from build123d import *

# Parameters (mm, degrees)
ESTRUSIONE_ESTRUSIONE3_DEPTH = 1.5


with BuildPart() as part:
    # Schizzo1 → Estrusione-Estrusione3 (new body, symmetric)
    with BuildSketch(Plane(origin=(0, 0, 0), x_dir=(0, 0, -1), z_dir=(1, 0, 0))):
        Polygon((-40.5, -20.5), (-37.5, -20.5), (-30.681818182, -20.5), (-30.681818182, -17.5), (-23.863636364, -17.5), (-23.863636364, -20.5), (-17.045454545, -20.5), (-17.045454545, -17.5), (-10.227272727, -17.5), (-10.227272727, -20.5), (-3.409090909, -20.5), (-3.409090909, -17.5), (3.409090909, -17.5), (3.409090909, -20.5), (10.227272727, -20.5), (10.227272727, -17.5), (17.045454545, -17.5), (17.045454545, -20.5), (23.863636364, -20.5), (23.863636364, -17.5), (30.681818182, -17.5), (30.681818182, -20.5), (37.5, -20.5), (40.5, -20.5), (40.5, -14.166666667), (37.5, -14.166666667), (37.5, -7.833333333), (40.5, -7.833333333), (40.5, -1.5), (37.5, -1.5), (37.5, 4.833333333), (40.5, 4.833333333), (40.5, 11.166666667), (37.5, 11.166666667), (37.5, 17.5), (-37.5, 17.5), (-37.5, 11.166666667), (-40.5, 11.166666667), (-40.5, 4.833333333), (-37.5, 4.833333333), (-37.5, -1.5), (-40.5, -1.5), (-40.5, -7.833333333), (-37.5, -7.833333333), (-37.5, -14.166666667), (-40.5, -14.166666667), align=None)
    extrude(amount=ESTRUSIONE_ESTRUSIONE3_DEPTH, both=True)


solid = part.part
Check sheet for the modelled part. Datum: model origin and axes. Units: mm. A direction names the side the tool comes from. Round coordinates to 2 decimals unless told otherwise and drop trailing zeros. Write each loop counter-clockwise with the first axis right and the second up, starting at its lowest first coordinate (ties: lowest second). Pieces come first, ordered by that corner, then holes. Notation, with made-up numbers: (89.5, -14) -> (102.5, -14) arc R22 ccw to (102.5, -8) -> close; hole circle Ø9 at (-10.75, -33.5). An arc over 180 degrees is marked (long way). Answer as CSV lines item,"result". Start each with the question number.
1) Material ranges on line 1 (Y direction, x = -0.2, z = 0.5); line 2 (Z direction, x = -0.3, y = 14), recorded low to high. Write a range as from..to.
2) Section check A-A on y = 2.5. Enter the section's corners in (x, z).
3) Release check for a two-part mould opening along Z. For faces 1 (the flat face through (0, -19, -23.864)), 2 (the flat face through (0, -19, -30.682)), 3 (the flat face through (0, 14, 37.5)), 4 (the flat face through (0, -14.167, 39)) record: pulls with the +Z half, pulls with the -Z half, needs draft (parallel to the pull), parting line crosses it, or undercut.
4) Tool access check on faces 5 (the flat face through (0, 11.167, 39)), 6 (the flat face through (0, -7.833, -39)), 7 (the flat face through (0, -19, 10.227)), 8 (the flat face through (0, -7.833, 39)), 9 (the flat face through (0, -20.5, 36)). Record the directions out of +Z, -Z, +X, -X, +Y, -Y that give a thin tool (end or side, any length) a straight path to the whole face; none if there is none.
5) Section check B-B on z = -13. Enter the section's corners in (x, y).
6) Go/stop test with flat-tipped pins: P1, Ø0.9, axis at x = -0.5, z = -39.5, coming from the +Y side; P2, Ø1.5, axis at x = 0.5, z = 0.5, coming from the -Y side. Record where each tip stops, or that it passes through.
Found:
1,line 1,"y = -17.5..17.5"
1,line 2,"z = -37.5..37.5"
2,outline,"(-1.5, -37.5) -> (1.5, -37.5) -> (1.5, 37.5) -> (-1.5, 37.5) -> close"
3,face 1,"undercut"
3,face 2,"undercut"
3,face 3,"pulls with the +Z half"
3,face 4,"needs draft"
4,face 5,"+Z, +X, -X, +Y"
4,face 6,"-Z, +X, -X"
4,face 7,"+X, -X, -Y"
4,face 8,"+Z, +X, -X"
4,face 9,"+Z, -Z, +X, -X, -Y"
5,outline,"(-1.5, -17.5) -> (1.5, -17.5) -> (1.5, 17.5) -> (-1.5, 17.5) -> close"
6,P1,"stops at y = 11.17"
6,P2,"stops at y = -17.5"
